Verification items for the finished model (mm, model axes). A direction names the side the tool comes from. Give positions to 0.01 mm unless a question says otherwise; leave off trailing zeros. Loops run counter-clockwise (first coordinate to the right, second up) from the corner with the lowest first, then second, coordinate; pieces in that order, holes last. Notation, with made-up numbers: (0, -14) - (10, -14) arc R16 cw to (10, 2) - close; hole circle Ø9 at (-15, 86). An arc over 180 degrees is marked (long way). One line per question, with ' | ' between items. Start each with the question number.
1. Mould release check, pull along X, two halves, no side actions. Record for faces 1 (the face through (9, 9, 3)), 2 (the face through (5, 2.5, 6)), 3 (the face through (7, 2, 9)): +X half, -X half, draft (parallel to the pull), parting line (faces both ways), or undercut.
2. Section check C-C, the plane z = 8. Enter the section's corners in (x, y).
3. Depth check by flat-ended pin: pin 1 Ø0.6 at (y, z) = (10.5, 4.5) entering from -X; pin 2 Ø3 at (x, z) = (2, 1) entering from +Y; pin 3 Ø1.5 at (x, z) = (4.5, 7.5) entering from +Y. Enter the tip coordinate at first touch or a pass-through.
4. Tool access check on faces 4 (the face through (4, 2, 6)), 5 (the face through (9, 6, 8)), 6 (the face through (0, 3, 1)), 7 (the face through (1, 6, 1)), 8 (the face through (2, 1, 6)). Record the directions out of +Z, -Z, +X, -X, +Y, -Y that give a thin tool (end or side, any length) a straight path to the whole face; none if there is none.
5. Thickness scan on line 1 along Y through (x, z) = (2.25, 4.5); line 2 along Y through (x, z) = (1, 1.5); line 3 along Z through (x, y) = (1.25, 1.5). Record the ranges inside material, lowest first. Write a range as from..to.
6. Section check B-B, the plane x = 7.5. Enter the section's corners in (y, z).
7. Section check A-A, the plane y = 3.75. Enter the section's corners in (x, z).
8. Section check D-D, the plane y = 10. Enter the section's corners in (x, z), then the cut area to 3 significant figures.
from build123d import *

# Parameters (mm, degrees)
BOSS_EXTRUDE1_DEPTH = 9
SKETCH2_W           = 5
SKETCH2_H           = 5
CUT_EXTRUDE1_DEPTH  = 3
CUT_EXTRUDE2_DEPTH  = 6


with BuildPart() as part:
    # Sketch1 → Boss-Extrude1 (new body)
    with BuildSketch(Plane.XY):
        with BuildLine():
            ThreePointArc((10, 6), (8.535533906, 9.535533906), (5, 11))
            Line((5, 11), (5, 9))
            ThreePointArc((5, 9), (7.121320344, 8.121320344), (8, 6))
            ThreePointArc((8, 6), (5, 3), (2, 6))
            Line((2, 6), (0, 6))
            Line((0, 6), (0, 0))
            Line((0, 0), (10, 0))
            Line((10, 0), (10, 6))
        make_face()
    extrude(amount=BOSS_EXTRUDE1_DEPTH)

    # Sketch2 → Cut-Extrude1 (cut)
    with BuildSketch(Plane.XY.offset(9)):
        with Locations((7.5, 8.5)):
            Rectangle(SKETCH2_W, SKETCH2_H)
    extrude(amount=-CUT_EXTRUDE1_DEPTH, mode=Mode.SUBTRACT)

    # Sketch3 → Cut-Extrude2 (cut)
    with BuildSketch(Plane.XY.offset(9)):
        Polygon((5, 3), (5, 2), (2, 2), (2, 0), (0, 0), (0, 6.616008908), (4.654546825, 5.714332837), align=None)
    extrude(amount=-CUT_EXTRUDE2_DEPTH, mode=Mode.SUBTRACT)


solid = part.part
Results list:
1) face 1: +X half | face 2: -X half | face 3: draft
2) outline: (2, 0) - (10, 0) - (10, 6) - (8, 6) arc R3 cw to (5, 3) - (5, 2) - (2, 2) - close
3) pin 1: x = 5 | pin 2: y = 6 | pin 3: y = 3.01
4) face 4: +Z, -X, +Y | face 5: +Z, +X, -X, +Y | face 6: +Z, -Z, -X, +Y, -Y | face 7: +Z, -Z, -X, +Y | face 8: +Z, -X, +Y, -Y
5) line 1: 0..2 | line 2: 0..6 | line 3: 0..3
6) outline: (0, 0) - (4.34, 0) - (4.34, 9) - (0, 9) - close; (7.66, 0) - (10.33, 0) - (10.33, 6) - (7.66, 6) - close
7) outline: (0, 0) - (3.02, 0) - (3.02, 3) - (0, 3) - close; (6.98, 0) - (10, 0) - (10, 9) - (6.98, 9) - close
8) outline: (5, 0) - (8, 0) - (8, 6) - (5, 6) - close | area: 18.0 mm²
